from build123d import *

# Parameters (mm, degrees)
SKETCH2_W           = 431.8
SKETCH2_H           = 812.8
BOSS_EXTRUDE1_DEPTH = 457.2
SKETCH3_W           = 406.4
SKETCH3_H           = 254
CUT_EXTRUDE1_DEPTH  = 38.1
SKETCH3_4_R         = 25.4
BOSS_EXTRUDE2_DEPTH = 76.2
SKETCH5_R           = 10
SKETCH5_W           = 76.2
SKETCH5_H           = 76.2
SKETCH5_W_2         = 180
SKETCH5_H_2         = 85
SKETCH5_W_3         = 72
BOSS_EXTRUDE3_DEPTH = 25.4
SKETCH6_W           = 609.6
SKETCH6_H           = 762
CUT_EXTRUDE2_DEPTH  = 798.57617818
SKETCH7_W           = 5.08
SKETCH7_H           = 762
BOSS_EXTRUDE4_DEPTH = 609.6
SKETCH8_W           = 609.6
SKETCH8_H           = 762
CUT_EXTRUDE3_DEPTH  = 798.57617818
SKETCH9_W           = 5.08
SKETCH9_H           = 762
BOSS_EXTRUDE5_DEPTH = 609.6
SKETCH10_W          = 220
SKETCH10_H          = 220
CUT_EXTRUDE5_DEPTH  = 25.4


with BuildPart() as part:
    # Sketch2 → Boss-Extrude1 (new, symmetric)
    with BuildSketch(Plane.XY):
        Rectangle(SKETCH2_W, SKETCH2_H)
    extrude(amount=BOSS_EXTRUDE1_DEPTH, both=True)

    # Sketch3 → Cut-Extrude1 (cut)
    with BuildSketch(Plane.XY.offset(457.2)):
        with Locations((0, 254)):
            Rectangle(SKETCH3_W, SKETCH3_H)
    extrude(amount=-CUT_EXTRUDE1_DEPTH, mode=Mode.SUBTRACT)

    # Sketch3<4> → Boss-Extrude2 (add)
    with BuildSketch(Plane.XY.offset(457.2)):
        with Locations(Location((165.1, -342.9, 0), (0, 0, 180))):
            Circle(SKETCH3_4_R)
        with Locations(Location((165.1, -254, 0), (0, 0, 180))):
            Circle(SKETCH3_4_R)
        with Locations(Location((165.1, -165.1, 0), (0, 0, 180))):
            Circle(SKETCH3_4_R)
        with Locations(Location((165.1, -76.2, 0), (0, 0, 180))):
            Circle(SKETCH3_4_R)
        with Locations(Location((165.1, 12.7, 0), (0, 0, 180))):
            Circle(SKETCH3_4_R)
    extrude(amount=BOSS_EXTRUDE2_DEPTH)

    # Sketch5 → Boss-Extrude3 (add)
    with BuildSketch(Plane.XY.offset(419.1)):
        with Locations((0, 355.6)):
            Circle(SKETCH5_R)
        with Locations((30, 355.6)):
            Circle(SKETCH5_R)
        with Locations((60, 355.6)):
            Circle(SKETCH5_R)
        with Locations((-152.4, 330.2)):
            Rectangle(SKETCH5_W, SKETCH5_H)
        with Locations((100.5, 182.2)):
            Rectangle(SKETCH5_W_2, SKETCH5_H_2)
        with Locations((100.5, 287.2)):
            Rectangle(SKETCH5_W_2, SKETCH5_H_2)
        with Locations((-154.5, 182.2)):
            Rectangle(SKETCH5_W_3, SKETCH5_H_2)
    extrude(amount=BOSS_EXTRUDE3_DEPTH)

    # Sketch6 → Cut-Extrude2 (cut, through all)
    with BuildSketch(Plane(origin=(215.9, 0, 0), x_dir=(0, 0, -1), z_dir=(1, 0, 0))):
        with Locations((127, 0)):
            Rectangle(SKETCH6_W, SKETCH6_H)
    extrude(amount=-CUT_EXTRUDE2_DEPTH, mode=Mode.SUBTRACT)

    # Sketch7 → Boss-Extrude4 (add)
    with BuildSketch(Plane.XY.offset(-431.8)):
        with Locations((213.36, 0)):
            Rectangle(SKETCH7_W, SKETCH7_H)
    extrude(amount=BOSS_EXTRUDE4_DEPTH)

    # Sketch8 → Cut-Extrude3 (cut, through all)
    with BuildSketch(Plane(origin=(215.9, 0, 0), x_dir=(0, 0, -1), z_dir=(1, 0, 0))):
        with Locations((127, 0)):
            Rectangle(SKETCH8_W, SKETCH8_H)
    extrude(amount=-CUT_EXTRUDE3_DEPTH, mode=Mode.SUBTRACT)

    # Sketch9 → Boss-Extrude5 (add)
    with BuildSketch(Plane.XY.offset(-431.8)):
        with Locations((-213.36, 0)):
            Rectangle(SKETCH9_W, SKETCH9_H)
    extrude(amount=BOSS_EXTRUDE5_DEPTH)

    # Sketch10 → Cut-Extrude5 (cut)
    with BuildSketch(Plane.ZY.offset(215.9)):
        with Locations((-262, 240)):
            Rectangle(SKETCH10_W, SKETCH10_H)
        with Locations((-262, 0)):
            Rectangle(SKETCH10_W, SKETCH10_H)
        with Locations((-262, -240)):
            Rectangle(SKETCH10_W, SKETCH10_H)
        with Locations((8, -240)):
            Rectangle(SKETCH10_W, SKETCH10_H)
        with Locations((8, 240)):
            Rectangle(SKETCH10_W, SKETCH10_H)
        with Locations((8, 0)):
            Rectangle(SKETCH10_W, SKETCH10_H)
    extrude(amount=-CUT_EXTRUDE5_DEPTH, mode=Mode.SUBTRACT)


solid = part.part
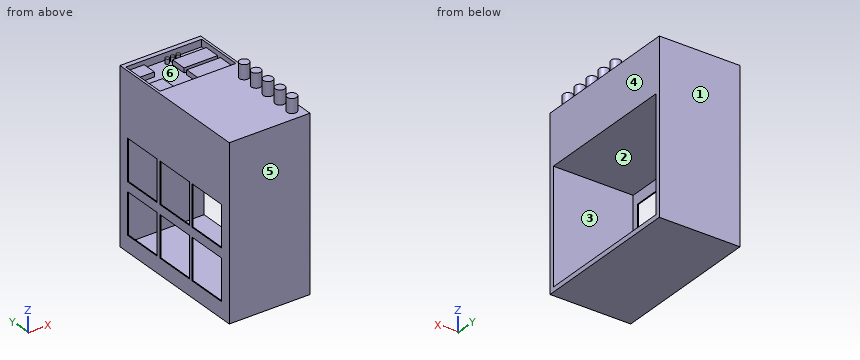
The model under review builds one solid part; all positions refer to its coordinate system, in mm. Face numbers are marked on the shaded views. A direction names the side the tool comes from. Round coordinates to 2 decimals unless told otherwise and drop trailing zeros. Loops run counter-clockwise (first coordinate to the right, second up) from the corner with the lowest first, then second, coordinate; pieces in that order, holes last. Notation, with made-up numbers: (77, 3.25) -> (94, 3.25) arc R29 ccw to (94, 31.25) -> close; hole circle Ø10 at (-0.5, 61.25). An arc over 180 degrees is marked (long way). One line per question, with ' | ' between items. Start each with the question number.
Item 1: Draft analysis for pull direction Y (two halves, no side actions). For the marked faces 3, 4, 5 and 6, state which applies: +Y half, -Y half, draft (parallel to the pull), parting line (faces both ways), or undercut.
Item 2: Add section C-C, the plane x = 120. Write out the cut boundary in (y, z), then the cut area to 3 significant figures.
Item 3: Add section A-A, the plane z = 23.5. Write out the cut boundary in (x, y), then the cut area to 3 significant figures.
Item 4: Add section B-B, the plane y = -76.2. Write out the cut boundary in (x, z), then the cut area to 3 significant figures.
Item 5: Machinability: for the marked faces 1 and 2, which of the approach directions +Z, -Z, +X, -X, +Y, -Y give a long, thin tool a straight path to every point of the face, cutting with its end or side? Answer none if there is none.
Item 6: For pin 1 (5 mm diameter, centred on x = 79, y = 131, fed in from +Z); pin 2 (5.5 mm diameter, centred on x = -213.5, y = 279.5, fed in from +Z), all flat-tipped, find the tip position at first contact; note any pin that passes through.
Item 7: Add section D-D, the plane y = 191.5. Write out the cut boundary in (x, z), then the cut area to 3 significant figures.
Item 8: Wall thickness on line 1 along Y through (x, z) = (137.5, 444); line 2 along Z through (x, y) = (-119, 106.5); line 3 along Y through (x, z) = (-125, 117.5): over which ranges is each line inside the solid? List them lowest first. Write a range as [from, to].
Return value:
1) face 3: undercut | face 4: draft | face 5: -Y half | face 6: undercut
2) outline: (-406.4, -457.2) -> (406.4, -457.2) -> (406.4, 457.2) -> (381, 457.2) -> (381, 419.1) -> (329.7, 419.1) -> (329.7, 444.5) -> (244.7, 444.5) -> (244.7, 419.1) -> (224.7, 419.1) -> (224.7, 444.5) -> (139.7, 444.5) -> (139.7, 419.1) -> (127, 419.1) -> (127, 457.2) -> (-406.4, 457.2) -> close; hole (-381, -431.8) -> (381, -431.8) -> (381, 177.8) -> (-381, 177.8) -> close | area: 273,000 mm2
3) outline: (-215.9, -406.4) -> (215.9, -406.4) -> (215.9, -381) -> (-210.82, -381) -> (-210.82, -350) -> (-215.9, -350) -> close; (-215.9, -130) -> (-210.82, -130) -> (-210.82, -110) -> (-215.9, -110) -> close; (-215.9, 110) -> (-210.82, 110) -> (-210.82, 130) -> (-215.9, 130) -> close; (-215.9, 350) -> (-210.82, 350) -> (-210.82, 381) -> (215.9, 381) -> (215.9, 406.4) -> (-215.9, 406.4) -> close | area: 22,500 mm2
4) outline: (-215.9, -457.2) -> (215.9, -457.2) -> (215.9, -431.8) -> (-210.82, -431.8) -> (-210.82, -372) -> (-215.9, -372) -> close; (-215.9, -152) -> (-210.82, -152) -> (-210.82, -102) -> (-215.9, -102) -> close; (-215.9, 118) -> (-210.82, 118) -> (-210.82, 177.8) -> (215.9, 177.8) -> (215.9, 457.2) -> (190.5, 457.2) -> (190.5, 533.4) -> (139.7, 533.4) -> (139.7, 457.2) -> (-215.9, 457.2) -> close | area: 136,000 mm2
5) face 1: +Z, -Z, +X, -X, +Y | face 2: +X
6) pin 1: stops at z = 419.1 | pin 2: stops at z = 457.2
7) outline: (-215.9, -457.2) -> (215.9, -457.2) -> (215.9, -431.8) -> (-210.82, -431.8) -> (-210.82, -372) -> (-215.9, -372) -> close; (-215.9, -152) -> (-210.82, -152) -> (-210.82, -102) -> (-215.9, -102) -> close; (-215.9, 118) -> (-210.82, 118) -> (-210.82, 177.8) -> (215.9, 177.8) -> (215.9, 457.2) -> (203.2, 457.2) -> (203.2, 419.1) -> (190.5, 419.1) -> (190.5, 444.5) -> (10.5, 444.5) -> (10.5, 419.1) -> (-118.5, 419.1) -> (-118.5, 444.5) -> (-190.5, 444.5) -> (-190.5, 419.1) -> (-203.2, 419.1) -> (-203.2, 457.2) -> (-215.9, 457.2) -> close | area: 123,000 mm2
8) line 1: y = [-406.4, 127], [139.7, 224.7], [244.7, 329.7], [381, 406.4] | line 2: z = [-457.2, -431.8], [177.8, 457.2] | line 3: y = [-406.4, -381], [381, 406.4]
